```python
from build123d import *

# Parameters (mm, degrees)
SKETCH1_W                                      = 90
SKETCH1_H                                      = 80
BOSS_EXTRUDE1_DEPTH                            = 50
SHELL1_T                                       = -2
SKETCH2_W                                      = 34.5
SKETCH2_H                                      = 24
CUT_EXTRUDE_DEPTH                              = 2
SKETCH3_W                                      = 15
SKETCH3_H                                      = 15
SKETCH3_W_2                                    = 6
SKETCH3_H_2                                    = 6
CUT_EXTRUDE2_DEPTH                             = 2
SKETCH4_R                                      = 2
BOSS_EXTRUDE3_DEPTH                            = 10
SKETCH7_W                                      = 7
SKETCH7_H                                      = 10
BOSS_EXTRUDE4_DEPTH                            = 4
BOSS_EXTRUDE4_DRAFT                            = 15
BOSS_EXTRUDE4_PROFILE_2_DEPTH                  = 4
BOSS_EXTRUDE4_PROFILE_2_DRAFT                  = 15
SKETCH11_W                                     = 8
SKETCH11_H                                     = 12
CUT_EXTRUDE3_DEPTH                             = 10
SKETCH12_W                                     = 20
SKETCH12_H                                     = 40
CUT_EXTRUDE4_DEPTH                             = 10
CSK_FOR_M3_OVAL_HEAD_MACHINE_SCREW1_AT_2_COUNT = 2
CSK_FOR_M3_OVAL_HEAD_MACHINE_SCREW1_AT_2_PITCH = 66.030296077
CSK_FOR_M3_OVAL_HEAD_MACHINE_SCREW1_AT_3_COUNT = 2
CSK_FOR_M3_OVAL_HEAD_MACHINE_SCREW1_AT_3_PITCH = 72.672209269


with BuildPart() as part:
    # Sketch1 → Boss-Extrude1 (new body)
    with BuildSketch(Plane.XY):
        Rectangle(SKETCH1_W, SKETCH1_H)
    extrude(amount=BOSS_EXTRUDE1_DEPTH)

    # Shell1
    shell1_openings = [part.faces().sort_by_distance(p)[0] for p in [
        (0, 0, 0),
    ]]
    offset(amount=SHELL1_T, openings=shell1_openings, kind=Kind.INTERSECTION)

    # Sketch2 → Cut-Extrude (cut)
    with BuildSketch(Plane.XY.offset(50)):
        with Locations((0.11, 19.1)):
            Rectangle(SKETCH2_W, SKETCH2_H)
    extrude(amount=-CUT_EXTRUDE_DEPTH, mode=Mode.SUBTRACT)

    # Sketch3 → Cut-Extrude2 (cut)
    with BuildSketch(Plane.XY.offset(50)):
        with Locations((23.7, -28.5)):
            Rectangle(SKETCH3_W, SKETCH3_H)
        with Locations((-23.7, -29)):
            Rectangle(SKETCH3_W, SKETCH3_H)
        with Locations((-7.25, -29.25)):
            Rectangle(SKETCH3_W_2, SKETCH3_H_2)
        with Locations((7.25, -29.25)):
            Rectangle(SKETCH3_W_2, SKETCH3_H_2)
    extrude(amount=-CUT_EXTRUDE2_DEPTH, mode=Mode.SUBTRACT)

    # Sketch4 → Boss-Extrude3 (add)
    with BuildSketch(Plane(origin=(0, 0, 48), x_dir=(-1, 0, 0), z_dir=(0, 0, -1))):
        with Locations((-34.5, -35)):
            Circle(SKETCH4_R)
        with Locations((0, -34)):
            Circle(SKETCH4_R)
        with Locations((-32.5, 31)):
            Circle(SKETCH4_R)
    extrude(amount=BOSS_EXTRUDE3_DEPTH)


with BuildPart() as boss_extrude4_tool:
    # Sketch7 → Boss-Extrude4 (with draft: the straight prism first)
    with BuildSketch(Plane.XZ.offset(40)):
        with Locations((-39, 42.5)):
            Rectangle(SKETCH7_W, SKETCH7_H)
    extrude(amount=BOSS_EXTRUDE4_DEPTH)
    # Boss-Extrude4: the draft: its side faces are tilted about the plane it starts from
    boss_extrude4_sides = [boss_extrude4_tool.faces().sort_by_distance(p)[0] for p in [
        (-42.5, -42, 42.5),
        (-39, -42, 37.5),
        (-35.5, -42, 42.5),
        (-39, -42, 47.5),
    ]]
    draft(boss_extrude4_sides, Plane.XZ.offset(40), BOSS_EXTRUDE4_DRAFT)


with BuildPart() as part_1:
    add(part.part)

    # Boss-Extrude4: add boss_extrude4_tool
    add(boss_extrude4_tool.part)


with BuildPart() as boss_extrude4_profile_2_tool:
    # Sketch7 → Boss-Extrude4 profile 2 (with draft: the straight prism first)
    with BuildSketch(Plane.XZ.offset(40)):
        with Locations((39, 42.5)):
            Rectangle(SKETCH7_W, SKETCH7_H)
    extrude(amount=BOSS_EXTRUDE4_PROFILE_2_DEPTH)
    # Boss-Extrude4 profile 2: the draft: its side faces are tilted about the plane it starts from
    boss_extrude4_profile_2_sides = [boss_extrude4_profile_2_tool.faces().sort_by_distance(p)[0] for p in [
        (35.5, -42, 42.5),
        (39, -42, 37.5),
        (42.5, -42, 42.5),
        (39, -42, 47.5),
    ]]
    draft(boss_extrude4_profile_2_sides, Plane.XZ.offset(40), BOSS_EXTRUDE4_PROFILE_2_DRAFT)


with BuildPart() as part_2:
    add(part_1.part)

    # Boss-Extrude4 profile 2: add boss_extrude4_profile_2_tool
    add(boss_extrude4_profile_2_tool.part)

    # Sketch11 → Cut-Extrude3 (cut)
    with BuildSketch(Plane.ZY.offset(45)):
        with Locations((41, -9)):
            Rectangle(SKETCH11_W, SKETCH11_H)
    extrude(amount=-CUT_EXTRUDE3_DEPTH, mode=Mode.SUBTRACT)

    # Sketch12 → Cut-Extrude4 (cut)
    with BuildSketch(Plane(origin=(45, 0, 0), x_dir=(0, 0, -1), z_dir=(1, 0, 0))):
        with Locations((-36, 0)):
            Rectangle(SKETCH12_W, SKETCH12_H)
    extrude(amount=-CUT_EXTRUDE4_DEPTH, mode=Mode.SUBTRACT)

    # Sketch14 → CSK for M3 Oval Head Machine Screw1 (revolve, cut)
    with BuildSketch(Plane(origin=(32.5, 31, 38), x_dir=(0, 1, 0), z_dir=(1, 0, 0))):
        Polygon((0, 0), (0, 11.021463052), (1.7, 10), (1.7, 1.45), (3.15, 0), align=None)
    csk_for_m3_oval_head_machine_screw1 = revolve(axis=Axis((32.5, 31, 31.65), (0, 0, 1)), mode=Mode.SUBTRACT)

    # CSK for M3 Oval Head Machine Screw1 at 2: CSK for M3 Oval Head Machine Screw1 ×2
    with Locations(*[Vector(0.030289126640769028, -0.9995411791453814, 0) * (i * CSK_FOR_M3_OVAL_HEAD_MACHINE_SCREW1_AT_2_PITCH) for i in range(1, CSK_FOR_M3_OVAL_HEAD_MACHINE_SCREW1_AT_2_COUNT)]):
        add(csk_for_m3_oval_head_machine_screw1, mode=Mode.SUBTRACT)

    # CSK for M3 Oval Head Machine Screw1 at 3: CSK for M3 Oval Head Machine Screw1 ×2
    with Locations(*[Vector(-0.447213595499958, -0.894427190999916, 0) * (i * CSK_FOR_M3_OVAL_HEAD_MACHINE_SCREW1_AT_3_PITCH) for i in range(1, CSK_FOR_M3_OVAL_HEAD_MACHINE_SCREW1_AT_3_COUNT)]):
        add(csk_for_m3_oval_head_machine_screw1, mode=Mode.SUBTRACT)


solid = part_2.part
```
Build history of the part. All positions in model axes, mm. A direction names the side the tool comes from. Give positions to 0.01 mm unless a question says otherwise; leave off trailing zeros. Order: outer loops, then holes, each group sorted by start corner. A loop starts at its lowest first (then second) coordinate and runs counter-clockwise, first axis right, second up. Notation, with made-up numbers: M -30.75,63.5 L 11.25,63.5 A16 cw 11.25,68.5 Z; hole C 37.5,33 d6. An arc over 180 degrees is marked long. Write item = value, one per line. Start each with the question number.
(1) Probe L1, parallel to X at y = 31, z = 45; L2, parallel to Y at x = 0, z = 46.25; L3, parallel to X at y = 4, z = 9. List the from-to ranges inside material, lowest first. Write a range as [from, to].
(2) Slice it at B-B on z = 16.5. Write the cut outline in (x, y).
(3) Two-plate mould, pull along X, no slides. Class faces 1 (the flat face through (4.25, -29, 49)), 2 (the flat face through (44, 0, 46)), 3 (the flat face through (-41.972, -41.972, 42.43)): released by +X, released by -X, zero draft, split by the parting line, or undercut.
(4) Slice it at C-C on y = -18.5. Write the cut outline in (x, z).
(5) Which spindle directions (+Z, -Z, +X, -X, +Y, -Y) get a long thin tool onto all of the face, cutting with end or side? Do faces 4 (the flat face through (-1, 1, 48)), 5 (the flat face through (0, 31.1, 49)), 6 (the flat face through (-44, -3, 41)). Say none if no direction does.
(6) Pin check, flat tips, straight feed: pin 1 Ø3 at (x, z) = (-20, 36) entering from -Y; pin 2 Ø14.5 at (y, z) = (6.5, 34.5) entering from +X; pin 3 Ø5 at (x, y) = (-1.5, 27) entering from +Z; pin 4 Ø1.5 at (x, y) = (-21.5, 30) entering from -Z. Stop position of each tip, or through.
(7) Slice it at A-A on x = 28. Write the cut outline in (y, z).
Responses:
q1.L1 = [-45, -43], [30.5, 30.8], [34.2, 34.5], [43, 45]
q1.L2 = [-40, -38], [-36, -35.7], [-32.3, -32], [38, 40]
q1.L3 = [-45, -43], [43, 45]
q2.outline = M -45,-40 L 45,-40 L 45,40 L -45,40 Z; hole M -43,-38 L 43,-38 L 43,38 L -43,38 Z
q3.face_1 = undercut
q3.face_2 = zero draft
q3.face_3 = released by -X
q4.outline = M -45,0 L -43,0 L -43,48 L 43,48 L 43,46 L 45,46 L 45,50 L -45,50 Z; M 43,0 L 45,0 L 45,26 L 43,26 Z
q5.face_4 = -Z
q5.face_5 = +Z, -Z
q5.face_6 = +X, -X
q6.pin_1 = -40
q6.pin_2 = -43
q6.pin_3 = through
q6.pin_4 = 48
q7.outline = M -40,0 L -38,0 L -38,48 L -36,48 L -36,50 L -40,50 Z; M -21,48 L 38,48 L 38,0 L 40,0 L 40,50 L -21,50 Z
